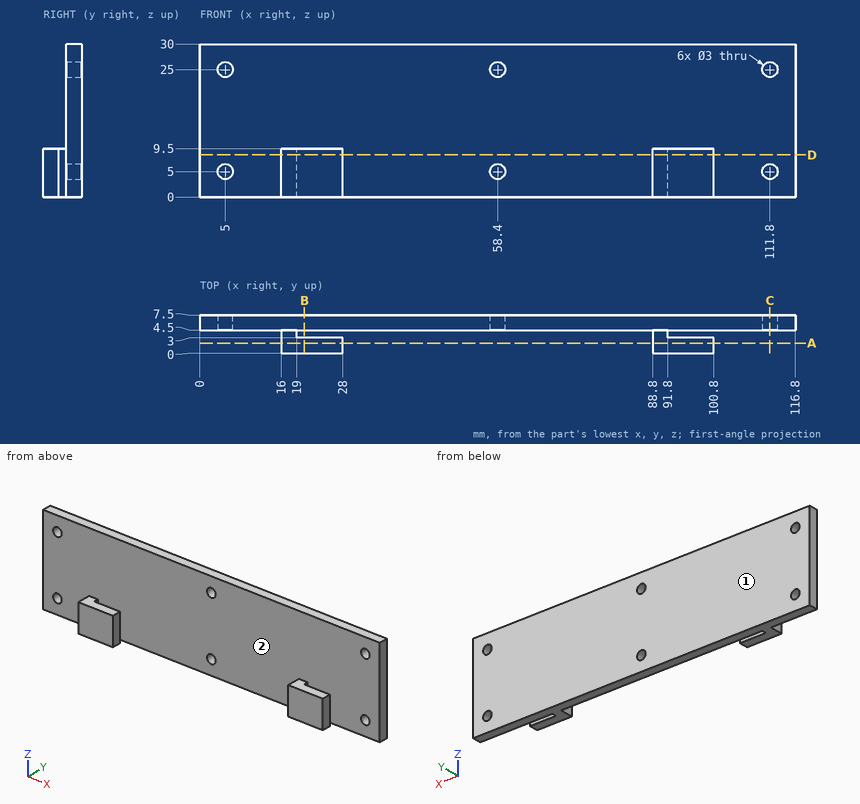
Geometry: see drawing. Coordinates: mm, zero at the bounding-box minimum. Give positions to 0.01 mm unless a question says otherwise; leave off trailing zeros. Write each loop counter-clockwise with the first axis right and the second up, starting at its lowest first coordinate (ties: lowest second). Pieces come first, ordered by that corner, then holes. Notation, with made-up numbers: M -10.5,6 L 26.5,6 A21 ccw 26.5,15 Z; hole C -18.75,58.5 d7. An arc over 180 degrees is marked long. Answer in a Markdown table with one row per item. Add a question column.
(1) Section D-D on z = 8.25. Return loops of the section in (x, y).
(2) Section B-B on x = 20.5. Return loops of the section in (y, z).
(3) First-contact query: pin 1 (1.5 mm diameter, centred on y = 2, z = 4, fed in from +X); pin 2 (6 mm diameter, centred on x = 50.5, z = 6.5, fed in from -Y). Flat tips, straight axial feed; report the tip coordinate or a pass-through.
(4) Mould query, pull axis X, two halves, no side actions, for the marked faces 1 and 2. Classes: +X half, -X half, draft (parallel to the pull), parting line (faces both ways), or undercut.
(5) Section C-C on x = 111.8. Return loops of the section in (y, z), and give its area (3 significant figures).
(6) Ray query, line 1 (Z direction, x = 111.8, y = 5.25); line 2 (X direction, y = 2.75, z = 5); line 3 (Y direction, x = 69, z = 16.75). Return the intervals inside material, ascending.
(7) Section A-A on y = 2. Return loops of the section in (x, z), and give its area (3 significant figures).
Result set:
| question | item | result |
|---|---|---|
| 1 | outline | M 0,4.5 L 16,4.5 L 16,0 L 28,0 L 28,3 L 19,3 L 19,4.5 L 88.8,4.5 L 88.8,0 L 100.8,0 L 100.8,3 L 91.8,3 L 91.8,4.5 L 116.8,4.5 L 116.8,7.5 L 0,7.5 Z |
| 2 | outline | M 0,0 L 3,0 L 3,9.5 L 0,9.5 Z; M 4.5,0 L 7.5,0 L 7.5,30 L 4.5,30 Z |
| 3 | pin 1 | stops at x = 100.8 |
| 3 | pin 2 | stops at y = 4.5 |
| 4 | face 1 | draft |
| 4 | face 2 | undercut |
| 5 | outline | M 4.5,0 L 7.5,0 L 7.5,3.5 L 4.5,3.5 Z; M 4.5,6.5 L 7.5,6.5 L 7.5,23.5 L 4.5,23.5 Z; M 4.5,26.5 L 7.5,26.5 L 7.5,30 L 4.5,30 Z |
| 5 | area | 72.0 mm^2 |
| 6 | line 1 | z = 0 to 3.5, 6.5 to 23.5, 26.5 to 30 |
| 6 | line 2 | x = 16 to 28, 88.8 to 100.8 |
| 6 | line 3 | y = 4.5 to 7.5 |
| 7 | outline | M 16,0 L 28,0 L 28,9.5 L 16,9.5 Z; M 88.8,0 L 100.8,0 L 100.8,9.5 L 88.8,9.5 Z |
| 7 | area | 228 mm^2 |
